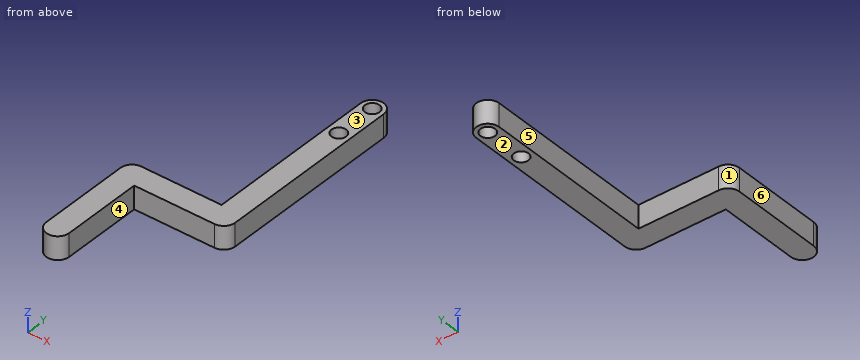
Autodesk Fusion 360 part; units mm, degrees
sketch "스케치1" plane through (0, 0, 0) normal (0, 0, 1) x (1, 0, 0)
  line L0 (-2.5, 25) -> (-2.5, -15)
  arc A0 (-2.5, -15) -> (2.5, -15) centre (0, -15) ccw
  line L1 (2.5, -15) -> (2.5, 25)
  arc A1 (2.5, 25) -> (-2.5, 25) centre (0, 25) ccw
  line L2 (0, 25) -> (0, -15) construction
  line L3 (0, -12.5) -> (-20, -12.5)
  arc A2 (-20, -12.5) -> (-20, -17.5) centre (-20, -15) ccw
  line L4 (-20, -17.5) -> (0, -17.5)
  arc A3 (0, -17.5) -> (0, -12.5) centre (0, -15) ccw
  line L5 (0, -15) -> (-20, -15) construction
  line L6 (-22.5, -15) -> (-22.5, -35)
  arc A4 (-22.5, -35) -> (-17.5, -35) centre (-20, -35) ccw
  line L7 (-17.5, -35) -> (-17.5, -15)
  arc A5 (-17.5, -15) -> (-22.5, -15) centre (-20, -15) ccw
  line L8 (-20, -15) -> (-20, -35) construction
  circle A6 centre (0, 25) radius 1.6
  line L9 (-10, 16) -> (11, 16)
  circle A7 centre (0, 16) radius 1.6
  dimension "d1" = 5
  dimension "d2" = 5
  dimension "d3" = 5
  dimension "d4" = 3.2
  dimension "d5" = 9
  dimension "d6" = 3.2
  dimension "d9" = 20
extrude "돌출1" add sketch "스케치1" along normal blind 5 contours L0 L1 A1 L9 A7 | L0 L1 L3 A3 L9 A7 | L0 A0 L3 A3 | L0 A0 L3 L4 L7 A5 | A2 L4 L7 A5 | A2 L4 L6 A4 L7
Model file for the job. Use its own axes, mm. Face numbers are marked on the shaded views. A direction names the side the tool comes from. Give positions to 0.01 mm unless a question says otherwise; leave off trailing zeros. Write each loop counter-clockwise with the first axis right and the second up, starting at its lowest first coordinate (ties: lowest second). Pieces come first, ordered by that corner, then holes. Notation, with made-up numbers: M 23.25,-2.5 L 78.25,-2.5 A32 cw 78.25,27.5 Z; hole C 83,60.5 d6. An arc over 180 degrees is marked long. Use a Markdown table: item, result.
1) Cut at B-B (y = 16). List the corners of the cut face in (x, z).
Responses:
| item | result |
|---|---|
| outline | M -2.5,0 L -1.6,0 L -1.6,5 L -2.5,5 Z; M 1.6,0 L 2.5,0 L 2.5,5 L 1.6,5 Z |
2) Drill centre lines: line 1 (Y direction, x = 0, z = 2.55); line 2 (Y direction, x = -0.75, z = 3.7); line 3 (X direction, y = 5.5, z = 2.7). Where is each one in solid material? Low to high. Write a range as from..to.
Responses:
| item | result |
|---|---|
| line 1 | y = -17.5..14.4, 17.6..23.4, 26.6..27.5 |
| line 2 | y = -17.5..14.59, 17.41..23.59, 26.41..27.38 |
| line 3 | x = -2.5..2.5 |
3) Pull direction Z, two halves, no side cores. Call the marked faces 1, 2 and 3: +Z half, -Z half, draft (parallel to the pull), parting line (faces both ways), or undercut.
Responses:
| item | result |
|---|---|
| face 1 | draft |
| face 2 | -Z half |
| face 3 | +Z half |
4) Cut at C-C (x = -15.75). List the corners of the cut face in (y, z).
Responses:
| item | result |
|---|---|
| outline | M -17.5,0 L -12.5,0 L -12.5,5 L -17.5,5 Z |
5) Tool access for the marked faces 4, 5 and 6: list every direction of +Z, -Z, +X, -X, +Y, -Y with a clear straight run to the whole face (end or side of a thin tool).
Responses:
| item | result |
|---|---|
| face 4 | +Z, -Z, +X, -Y |
| face 5 | +Z, -Z, -X, +Y |
| face 6 | +Z, -Z, -X, +Y, -Y |
6) Pin check, flat tips, straight feed: pin 1 (1.5 mm diameter, centred on y = -7.5, z = 2.5, fed in from -X); pin 2 (5 mm diameter, centred on x = 0, y = 25, fed in from +Z); pin 3 (1.5 mm diameter, centred on x = -9, z = 1.5, fed in from -Y). Stop position of each tip, or through.
Responses:
| item | result |
|---|---|
| pin 1 | stops at x = -2.5 |
| pin 2 | stops at z = 5 |
| pin 3 | stops at y = -17.5 |
7) Cut at A-A (z = 1.35). List the corners of the cut face in (x, y).
Responses:
| item | result |
|---|---|
| outline | M -22.5,-35 A2.5 ccw -17.5,-35 L -17.5,-17.5 L 0,-17.5 A2.5 ccw 2.5,-15 L 2.5,25 A2.5 ccw -2.5,25 L -2.5,-12.5 L -20,-12.5 A2.5 ccw -22.5,-15 Z; hole C 0,16 d3.2; hole C 0,25 d3.2 |
8) Cut at D-D (y = -2.5). List the corners of the cut face in (x, z), and give its area (3 significant figures).
Responses:
| item | result |
|---|---|
| outline | M -2.5,0 L 2.5,0 L 2.5,5 L -2.5,5 Z |
| area | 25.0 mm2 |
